The listing builds one solid part. Answer for the finished solid, in the listing's coordinates (mm). Coordinates: 2 decimals unless noted, no trailing zeros. Write each loop counter-clockwise with the first axis right and the second up, starting at its lowest first coordinate (ties: lowest second). Pieces come first, ordered by that corner, then holes.
(1) Straight lines are drawn through the part: line 1 (X direction, y = 2.9, z = 19.5); line 2 (Z direction, x = 88.5, y = 0.95); line 3 (X direction, y = 1.2, z = 26). For each, find the intervals that lie inside material, in ascending order.
(2) The part is cut by section C-C on x = 28. Determine the outline of the cut face in (y, z), plus the area to 3 significant figures.
(3) The part is cut by section A-A on z = 18.5. Determine the outline of the cut face in (x, y), plus the area to 3 significant figures.
(4) Given P1, Ø1, axis at x = -1.5, y = 1, coming from the -Z side; P2, Ø0.6, axis at x = -1, y = 1.5, coming from the +Z side; P3, Ø1.5, axis at y = 1, z = 31, coming from the +X side; P4, Ø3.5, axis at x = 0, z = 63, coming from the -Y side, each flat-ended and moving along its own axis, determine where each tip first touches the part or whether it passes through.
(5) The part is cut by section B-B on y = 2.45. Give the number of separate pieces and of enclosed holes in the cut face, plus the area to 3 significant figures.
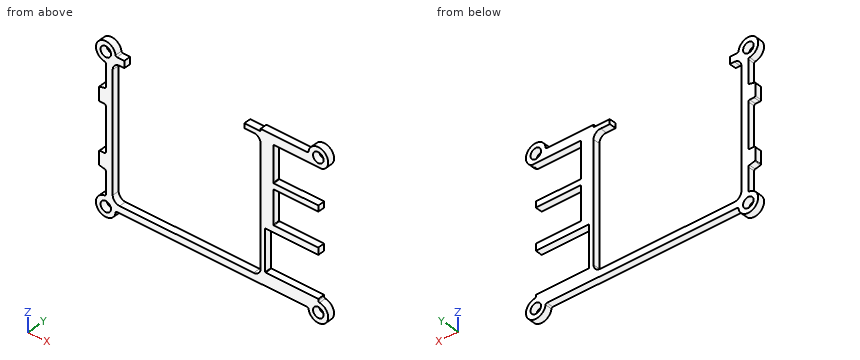
from build123d import *

# Parameters (mm, degrees)
SKETCH1_R           = 2.265
BOSS_EXTRUDE1_DEPTH = 3
SKETCH2_W           = 6.5
SKETCH2_H           = 20
CUT_EXTRUDE1_DEPTH  = 3
BOSS_EXTRUDE2_DEPTH = 3
CUT_EXTRUDE2_DEPTH  = 3
SKETCH5_W           = 3
SKETCH5_H           = 20
BOSS_EXTRUDE3_DEPTH = 3
SKETCH6_W           = 27.010134686
SKETCH6_H           = 17.9
CUT_EXTRUDE3_DEPTH  = 3
SKETCH7_W           = 19.5
SKETCH7_H           = 14.6
CUT_EXTRUDE4_DEPTH  = 3
SKETCH8_W           = 19.5
SKETCH8_H           = 15.6
CUT_EXTRUDE5_DEPTH  = 3
SKETCH9_W           = 2.019620965
SKETCH9_H           = 0.574286347
CUT_EXTRUDE6_DEPTH  = 3
SKETCH10_W          = 52
SKETCH10_H          = 3
CUT_EXTRUDE7_DEPTH  = 3
SKETCH11_W          = 7
SKETCH11_H          = 1
CUT_EXTRUDE8_DEPTH  = 3
FILLET1_R           = 0.6
FILLET2_R           = 0.2


with BuildPart() as part:
    # Sketch1 → Boss-Extrude1 (new body)
    with BuildSketch(Plane(origin=(0, 0, 0), x_dir=(1, 0, 0), z_dir=(0, 1, 0))):
        with BuildLine():
            Line((4.265, 0), (87.735, 0))
            ThreePointArc((87.735, 0), (95.015810422, 3.015810422), (92, -4.265))
            Line((92, -4.265), (92, -58.735))
            ThreePointArc((92, -58.735), (95.015810422, -66.015810422), (87.735, -63))
            Line((87.735, -63), (4.265, -63))
            ThreePointArc((4.265, -63), (-3.015810422, -66.015810422), (0, -58.735))
            Line((0, -58.735), (0, -4.265))
            ThreePointArc((0, -4.265), (-3.015810422, 3.015810422), (4.265, 0))
        make_face()
        with Locations(Location((0, 0, 0), (0, 0, 270))):
            Circle(SKETCH1_R, mode=Mode.SUBTRACT)
        with Locations(Location((92, 0, 0), (0, 0, 270))):
            Circle(SKETCH1_R, mode=Mode.SUBTRACT)
        with Locations(Location((92, -63, 0), (0, 0, 270))):
            Circle(SKETCH1_R, mode=Mode.SUBTRACT)
        with Locations(Location((0, -63, 0), (0, 0, 270))):
            Circle(SKETCH1_R, mode=Mode.SUBTRACT)
    extrude(amount=BOSS_EXTRUDE1_DEPTH)

    # Sketch2 → Cut-Extrude1 (cut)
    with BuildSketch(Plane(origin=(0, 3, 0), x_dir=(1, 0, 0), z_dir=(0, 1, 0))):
        with Locations((3.25, -31.5)):
            Rectangle(SKETCH2_W, SKETCH2_H)
    extrude(amount=-CUT_EXTRUDE1_DEPTH, mode=Mode.SUBTRACT)

    # Sketch3 → Boss-Extrude2 (add)
    with BuildSketch(Plane(origin=(0, 3, 0), x_dir=(1, 0, 0), z_dir=(0, 1, 0))):
        with BuildLine():
            Line((-2.7, -15.5), (0, -14.9))
            Line((0, -14.9), (0, -21.5))
            Line((0, -21.5), (-2.5, -21.5))
            ThreePointArc((-2.5, -21.5), (-2.853553391, -21.353553391), (-3, -21))
            Line((-3, -21), (-3, -15.8))
            ThreePointArc((-3, -15.8), (-2.912132034, -15.587867966), (-2.7, -15.5))
        make_face()
        with BuildLine():
            Line((-3, -42), (-3, -47.2))
            ThreePointArc((-3, -47.2), (-2.912132034, -47.412132034), (-2.7, -47.5))
            Line((-2.7, -47.5), (0, -48.1))
            Line((0, -48.1), (0, -41.5))
            Line((0, -41.5), (-2.5, -41.5))
            ThreePointArc((-2.5, -41.5), (-2.853553391, -41.646446609), (-3, -42))
        make_face()
    extrude(amount=-BOSS_EXTRUDE2_DEPTH)

    # Sketch4 → Cut-Extrude2 (cut)
    with BuildSketch(Plane(origin=(0, 3, 0), x_dir=(1, 0, 0), z_dir=(0, 1, 0))):
        with BuildLine():
            Line((6, -3), (64, -3))
            ThreePointArc((64, -3), (66.121320344, -3.878679656), (67, -6))
            Line((67, -6), (67, -57))
            ThreePointArc((67, -57), (66.121320344, -59.121320344), (64, -60))
            Line((64, -60), (6, -60))
            ThreePointArc((6, -60), (3.878679656, -59.121320344), (3, -57))
            Line((3, -57), (3, -6))
            ThreePointArc((3, -6), (3.878679656, -3.878679656), (6, -3))
        make_face()
    extrude(amount=-CUT_EXTRUDE2_DEPTH, mode=Mode.SUBTRACT)

    # Sketch5 → Boss-Extrude3 (add)
    with BuildSketch(Plane(origin=(0, 3, 0), x_dir=(1, 0, 0), z_dir=(0, 1, 0))):
        with Locations((1.5, -31.5)):
            Rectangle(SKETCH5_W, SKETCH5_H)
    extrude(amount=-BOSS_EXTRUDE3_DEPTH)

    # Sketch6 → Cut-Extrude3 (cut)
    with BuildSketch(Plane(origin=(0, 3, 0), x_dir=(1, 0, 0), z_dir=(0, 1, 0))):
        with Locations((82.505067343, -14.45)):
            Rectangle(SKETCH6_W, SKETCH6_H)
    extrude(amount=-CUT_EXTRUDE3_DEPTH, mode=Mode.SUBTRACT)

    # Sketch7 → Cut-Extrude4 (cut)
    with BuildSketch(Plane(origin=(0, 3, 0), x_dir=(1, 0, 0), z_dir=(0, 1, 0))):
        with Locations((82.25, -33.7)):
            Rectangle(SKETCH7_W, SKETCH7_H)
    extrude(amount=-CUT_EXTRUDE4_DEPTH, mode=Mode.SUBTRACT)

    # Sketch8 → Cut-Extrude5 (cut)
    with BuildSketch(Plane(origin=(0, 3, 0), x_dir=(1, 0, 0), z_dir=(0, 1, 0))):
        with Locations((82.25, -51.3)):
            Rectangle(SKETCH8_W, SKETCH8_H)
    extrude(amount=-CUT_EXTRUDE5_DEPTH, mode=Mode.SUBTRACT)

    # Sketch9 → Cut-Extrude6 (cut)
    with BuildSketch(Plane(origin=(0, 3, 0), x_dir=(1, 0, 0), z_dir=(0, 1, 0))):
        with Locations((93.009810483, -58.812856827)):
            Rectangle(SKETCH9_W, SKETCH9_H)
    extrude(amount=-CUT_EXTRUDE6_DEPTH, mode=Mode.SUBTRACT)

    # Sketch10 → Cut-Extrude7 (cut)
    with BuildSketch(Plane(origin=(0, 3, 0), x_dir=(1, 0, 0), z_dir=(0, 1, 0))):
        with Locations((34, -61.5)):
            Rectangle(SKETCH10_W, SKETCH10_H)
    extrude(amount=-CUT_EXTRUDE7_DEPTH, mode=Mode.SUBTRACT)

    # Sketch11 → Cut-Extrude8 (cut)
    with BuildSketch(Plane(origin=(0, 3, 0), x_dir=(1, 0, 0), z_dir=(0, 1, 0))):
        with Locations((63.5, -62.5)):
            Rectangle(SKETCH11_W, SKETCH11_H)
    extrude(amount=-CUT_EXTRUDE8_DEPTH, mode=Mode.SUBTRACT)

    # Fillet1
    fillet1_edges = [part.edges().sort_by_distance(p)[0] for p in [
        (0, 1.5, 41.5),
        (92, 1.5, 4.265),
        (0, 1.5, 21.5),
        (87.735, 1.5, 63),
        (4.265, 1.5, 63),
        (0, 1.5, 58.735),
        (0, 1.5, 4.265),
        (4.265, 1.5, 0),
        (87.735, 1.5, 0),
        (93.726332818, 1.5, 59.1),
        (0, 1.5, 14.9),
        (0, 1.5, 48.1),
    ]]
    fillet(fillet1_edges, radius=FILLET1_R)

    # Fillet2
    fillet2_edges = [part.edges().sort_by_distance(p)[0] for p in [
        (69, 1.5, 5.5),
        (69, 1.5, 23.4),
        (72.5, 1.5, 41),
        (72.5, 1.5, 26.4),
        (72.5, 1.5, 59.1),
        (72.5, 1.5, 43.5),
        (67, 1.5, 62),
    ]]
    fillet(fillet2_edges, radius=FILLET2_R)


solid = part.part
Model answer:
1. line 1: x = -3 to 3, 67 to 69
1. line 2: z = -2.44 to 5.5, 23.4 to 26.4, 41 to 43.5, 59.1 to 65.44
1. line 3: x = 0 to 3, 67 to 92
2. outline: (0, 0) - (3, 0) - (3, 3) - (0, 3) - close
2. area: 9.00 mm2
3. outline: (-3, 0) - (3, 0) - (3, 3) - (-3, 3) - close; (67, 0) - (69, 0) - (69, 3) - (67, 3) - close
3. area: 24.0 mm2
4. P1: stops at z = -4.15
4. P2: stops at z = 67.21
4. P3: stops at x = 72.5
4. P4: passes through
5. separate pieces: 1
5. enclosed holes: 4
5. area: 1,140 mm2
